Part print with two shaded views. Sizes in mm from the minimum x, y, z corner. Give positions to 0.01 mm unless a question says otherwise; leave off trailing zeros. Write each loop counter-clockwise with the first axis right and the second up, starting at its lowest first coordinate (ties: lowest second). Pieces come first, ordered by that corner, then holes. Notation, with made-up numbers: (85, 10.25) - (128, 10.25) arc R33 cw to (128, 45.25) - close; hole circle Ø5 at (57, -16.5). An arc over 180 degrees is marked (long way). Answer as a JSON object with one key per item and string values. Group by question number.
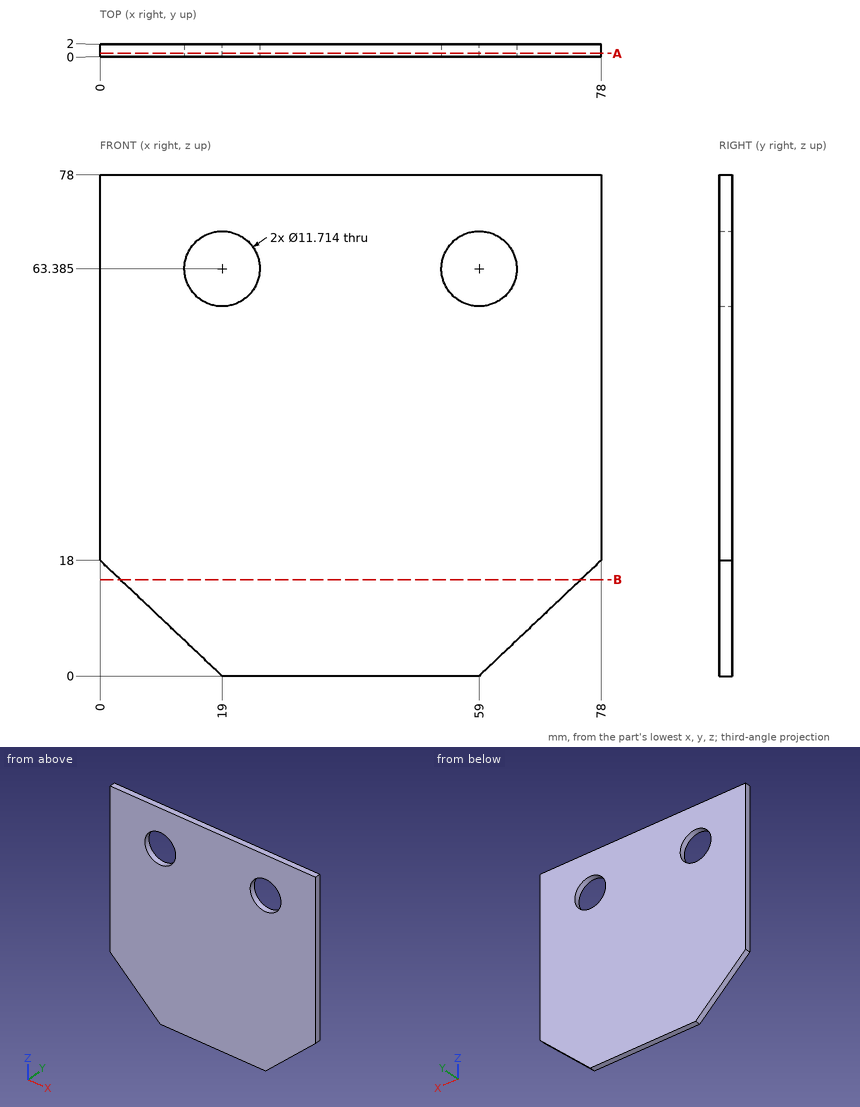
1) Drop flat-ended pins along their axis: P1, Ø10.5, axis at x = 59, z = 63.38, coming from the +Y side; P2, Ø1, axis at y = 1, z = 17, coming from the -X side. Give the stop position or say it passes through.
2) Drill centre lines: line 1 along Z through (x, y) = (59, 0.75); line 2 along X through (y, z) = (0.15, 68) (1 decimal); line 3 along Z through (x, y) = (62.5, 0.8) (1 decimal). Where is each one in solid material? Low to high. Write a range as from..to.
3) Saw through at A-A (y = 0.55). List the corners of the cut face in (x, z) (1 decimal), and give its area (3 significant figures).
4) Saw through at B-B (z = 15). List the corners of the cut face in (x, y), and give its area (3 significant figures).
Checks:
{
 "1": {"P1": "through", "P2": "x = 0.53"},
 "2": {"line 1": "0..57.53, 69.24..78", "line 2": "0..15.4, 22.6..55.4, 62.6..78", "line 3": "3.3..58.7, 68.1..78"},
 "3": {"outline": "(0, 18) - (19, 0) - (59, 0) - (78, 18) - (78, 78) - (0, 78) - close; hole circle Ø11.7 at (19, 63.4); hole circle Ø11.7 at (59, 63.4)", "area": "5,530 mm2"},
 "4": {"outline": "(3.17, 0) - (74.83, 0) - (74.83, 2) - (3.17, 2) - close", "area": "143 mm2"}
}
